Design review of the part built by this model. Coordinates are the model's own, in mm. A direction names the side the tool comes from. Give positions to 0.01 mm unless a question says otherwise; leave off trailing zeros. Loops run counter-clockwise (first coordinate to the right, second up) from the corner with the lowest first, then second, coordinate; pieces in that order, holes last.
from build123d import *

# Parameters (mm, degrees)
F0_W     = 50.8
F0_H     = 25.4
F1_DEPTH = 25.4
F2_W     = 26.06531
F2_H     = 25.4
F3_DEPTH = 25.4
F5_DEPTH = 50.8
F7_DEPTH = 25.4


with BuildPart() as f1:
    # F0 (on Top) → F1 (new body)
    with BuildSketch(Plane.XY):
        with Locations((-25.4, 12.7)):
            Rectangle(F0_W, F0_H)
    extrude(amount=F1_DEPTH)

    # F2 (on Top) → F3 (join)
    with BuildSketch(Plane.XY):
        with Locations((-13.032655, -12.7)):
            Rectangle(F2_W, F2_H)
    extrude(amount=F3_DEPTH)

    # F4 (on face) → F5 (join)
    with BuildSketch(Plane.XY.offset(25.4)):
        Polygon((0, -25.4), (0, 25.4), (-50.8, 25.4), (-50.8, 0), (-26.06531, 0), (-26.06531, -25.4), align=None)
    extrude(amount=F5_DEPTH)

    # F6 (on face) → F7 (join)
    with BuildSketch(Plane.YZ):
        Polygon((-55.88, 0), (-25.4, 0), (25.4, 0), (25.4, 76.2), (-23.200989, 76.2), (-55.88, 76.2), align=None)
    extrude(amount=F7_DEPTH)


solid = f1.part
Q1. Take a section at B-B (x = -46). Give the boundary of the cut face in (y, z), plus the area to 3 significant figures.
Results:
outline: (0, 0) - (25.4, 0) - (25.4, 76.2) - (0, 76.2) - close
area: 1,940 mm2
Q2. Insertion check: pin 1 (1 mm diameter, centred on y = -13.5, z = 67.5, fed in from -X); pin 2 (8 mm diameter, centred on x = -20, z = 35, fed in from -Y). Each pin has a flat end and moves straight along its axis. Give the tip position at first contact, or say it passes through.
Results:
pin 1: stops at x = -26.07
pin 2: stops at y = -25.4
Q3. Take a section at A-A (z = 26.5). Give the boundary of the cut face in (x, y), plus the area to 3 significant figures.
Results:
outline: (-50.8, 0) - (-26.07, 0) - (-26.07, -25.4) - (0, -25.4) - (0, -55.88) - (25.4, -55.88) - (25.4, 25.4) - (-50.8, 25.4) - close
area: 4,020 mm2
Q4. Wall thickness on line 1 (Y direction, x = -1, z = 6); line 2 (X direction, y = -9, z = 29.5); line 3 (X direction, y = -48, z = 65.5): over which ranges is each line inside the solid? List them lowest first.
Results:
line 1: y = -25.4 to 25.4
line 2: x = -26.07 to 25.4
line 3: x = 0 to 25.4
Q5. Tool access review of faces 1 (the face through (-26.065, -13, 38)), 2 (the face through (-13, 25.4, 38)): name each direction out of +Z, -Z, +X, -X, +Y, -Y from which nothing blocks a thin tool from reaching the whole face with its end or side.
Results:
face 1: +Z, -Z, -X, -Y
face 2: +Z, -Z, +X, -X, +Y
